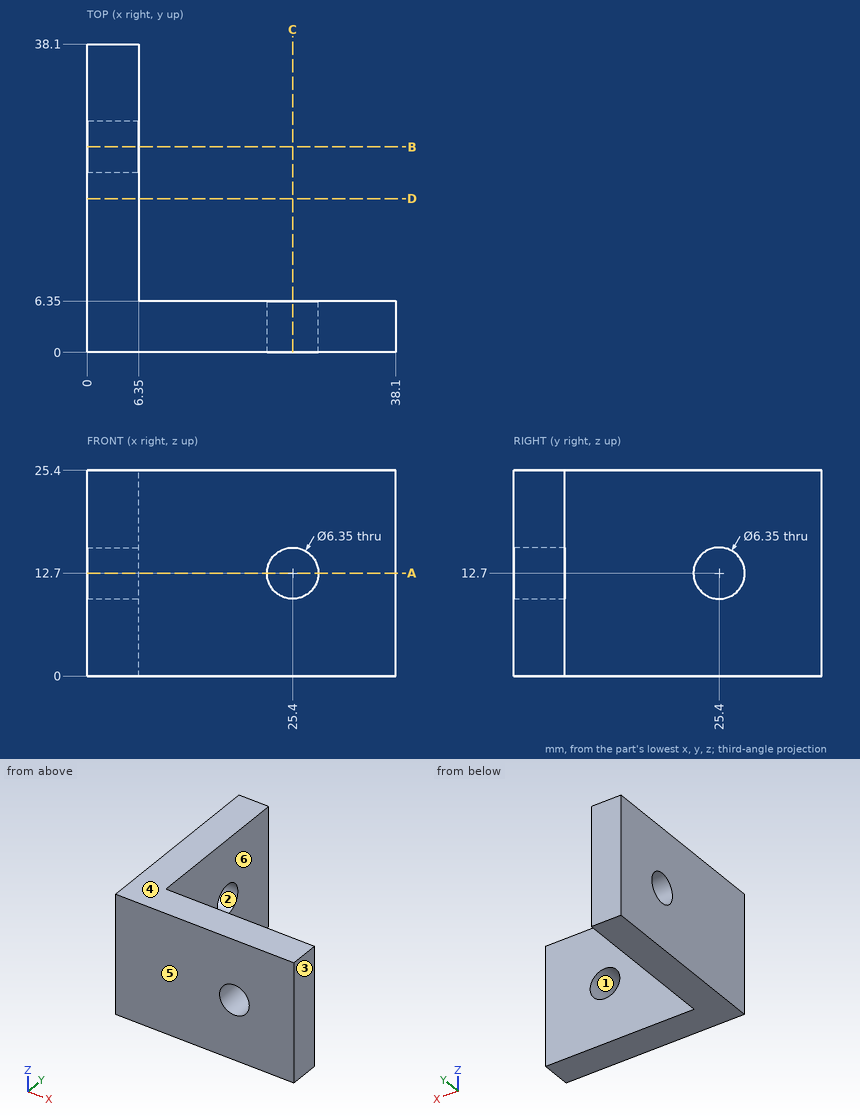
Can you work these out from the drawing? Everything is in mm from the part's minimum corner. A direction names the side the tool comes from. Round coordinates to 2 decimals unless told otherwise and drop trailing zeros. Loops run counter-clockwise (first coordinate to the right, second up) from the corner with the lowest first, then second, coordinate; pieces in that order, holes last.
1. If we section it at D-D on y = 19: Write out the boundary of the cut face in (x, z).
Answer list:
outline: (0, 0) - (6.35, 0) - (6.35, 25.4) - (0, 25.4) - close
2. We'd pull the mould along Z, two halves only. Please class the marked faces 1, 2, 3 and 4: +Z half, -Z half, draft (parallel to the pull), parting line (faces both ways), or undercut.
Answer list:
face 1: undercut
face 2: undercut
face 3: draft
face 4: +Z half
3. Which directions (+Z, -Z, +X, -X, +Y, -Y) give clear straight access to the entire face, cutting with the end or side of a thin tool? Please do the marked faces 5 and 6.
Answer list:
face 5: +Z, -Z, +X, -X, -Y
face 6: +Z, -Z, +X, +Y
4. If we section it at B-B on y = 25.4: Write out the boundary of the cut face in (x, z) (3 decimals), plus the area to 3 significant figures.
Answer list:
outline: (0, 0) - (6.35, 0) - (6.35, 9.525) - (0, 9.525) - close; (0, 15.875) - (6.35, 15.875) - (6.35, 25.4) - (0, 25.4) - close
area: 121 mm2
5. If I drill on line 1 along Z through (x, y) = (2.75, 25.4) (3 decimals); line 2 along X through (y, z) = (4.5, 12.7) (3 decimals); line 3 along X through (y, z) = (10, 7.5), over which ranges is the centre line in solid material (lowest first)?
Answer list:
line 1: z = 0 to 9.525, 15.875 to 25.4
line 2: x = 0 to 22.225, 28.575 to 38.1
line 3: x = 0 to 6.35
6. If we section it at A-A on z = 12.7: Write out the boundary of the cut face in (x, y) (3 decimals).
Answer list:
outline: (0, 0) - (22.225, 0) - (22.225, 6.35) - (6.35, 6.35) - (6.35, 22.225) - (0, 22.225) - close; (0, 28.575) - (6.35, 28.575) - (6.35, 38.1) - (0, 38.1) - close; (28.575, 0) - (38.1, 0) - (38.1, 6.35) - (28.575, 6.35) - close
7. For P1, Ø12, axis at x = 16.5, z = 9.5, coming from the +Y side; P2, Ø1.5, axis at y = 30, z = 6.5, coming from the +X side, each with a flat end and sliding along its axis, tell me the tip position at first contact or that it passes through.
Answer list:
P1: stops at y = 6.35
P2: stops at x = 6.35
